Autodesk Inventor part; units mm, degrees
ref_plane "YZ Plane" through (0, 0, 0) normal (1, 0, 0) x (0, 1, 0)
ref_plane "XZ Plane" through (0, 0, 0) normal (0, 1, 0) x (-1, 0, 0)
ref_plane "XY Plane" through (0, 0, 0) normal (0, 0, 1) x (1, 0, 0)
sketch "草图1" plane through (0, 0, 0) normal (0, 1, 0) x (-1, 0, 0)
  line L0 (0, 0) -> (83, 0)
  line L1 (83, 0) -> (83, -124)
  line L2 (83, -124) -> (0, -124)
  line L3 (0, -124) -> (0, 0)
  line L4 (-2, 2) -> (85, 2)
  line L5 (85, 2) -> (85, -126)
  line L6 (85, -126) -> (-2, -126)
  line L7 (-2, -126) -> (-2, 2)
  dimension "d0" = 83
  dimension "d1" = 124
  dimension "d2" = 2
  dimension "d3" = 2
  dimension "d4" = 2
extrude "拉伸1" add sketch "草图1" along normal blind 5 contours L0 L1 L2 L3 | L4 L5 L6 L7
sketch "草图2" plane through (-85, 0, 2) normal (0, 0, 1) x (1, 0, 0)
  line L0 (0, 0) -> (87, 0)
  line L1 (87, 0) -> (87, 5)
  line L2 (0, 5) -> (87, 5)
  line L3 (0, 0) -> (0, 5)
  line L4 (85, 0) -> (2, 0)
  line L5 (8, 0) -> (79, 0)
  line L6 (79, 0) -> (79, 2.5)
  line L7 (79, 2.5) -> (8, 2.5)
  line L8 (8, 2.5) -> (8, 0)
  point P0 (79, 1.25)
  dimension "d8" = 8
  dimension "d9" = 8
extrude "拉伸2" cut sketch "草图2" against normal through all contours L8 L7 L6 L0
sketch "草图3" plane through (2, 0, 2) normal (1, 0, 0) x (0, 0, -1)
  line L0 (2, 0) -> (126, 0)
  line L1 (8, 0) -> (120, 0)
  line L2 (120, 0) -> (120, 2.5)
  line L3 (120, 2.5) -> (8, 2.5)
  line L4 (8, 2.5) -> (8, 0)
  line L5 (0, 0) -> (0, 5)
  line L6 (128, 0) -> (128, 5)
  line L7 (0, 5) -> (128, 5)
  point P0 (8, 1.25)
  point P1 (120, 1.25)
  dimension "d12" = 8
  dimension "d13" = 8
  dimension "d14" = 2.5
extrude "拉伸3" cut sketch "草图3" against normal through all
sketch "草图4" plane through (0, 0, 0) normal (0, -1, 0) x (1, 0, 0)
  line L0 (-6, -6) -> (2, -6)
  line L1 (2, 2) -> (2, -6)
  line L2 (-6, 2) -> (2, 2)
  line L3 (-6, 2) -> (-6, -6)
  line L4 (-6, -6) -> (2, -6)
  line L5 (-77, -126) -> (-77, -118)
  line L6 (-85, 2) -> (-77, 2)
  line L7 (-85, -6) -> (-85, 2)
  line L8 (2, -118) -> (-6, -118)
  line L9 (-85, -126) -> (-85, -118)
  line L10 (-77, -126) -> (-85, -126)
  line L11 (-77, -126) -> (-77, -118)
  line L12 (2, -118) -> (-6, -118)
  line L13 (-6, 2) -> (-6, -6)
  line L14 (2, -126) -> (-6, -126)
  line L15 (2, -118) -> (2, -126)
  line L16 (-6, -118) -> (-6, -126)
  line L17 (-77, -118) -> (-85, -118)
  line L18 (-85, -126) -> (-85, -118)
  line L19 (-77, -126) -> (-85, -126)
  line L20 (-77, -126) -> (-77, -118)
  line L21 (-6, -6) -> (2, -6)
  line L22 (2, 2) -> (2, -6)
  line L23 (-6, 2) -> (2, 2)
  line L24 (-6, -6) -> (2, -6)
  line L25 (-85, 2) -> (-77, 2)
  line L26 (-85, -6) -> (-85, 2)
  line L27 (-6, 2) -> (-6, -6)
  line L28 (2, -126) -> (-6, -126)
  line L29 (2, -118) -> (2, -126)
  line L30 (-77, -118) -> (-85, -118)
  line L31 (-77, -6) -> (-77, 2)
  line L32 (-85, -6) -> (-77, -6)
  line L33 (2, -118) -> (-6, -118)
  line L34 (-85, -126) -> (-85, -118)
  line L35 (-77, -126) -> (-85, -126)
  line L36 (-77, -6) -> (-77, 2)
  line L37 (2, 2) -> (2, -6)
  line L38 (-6, 2) -> (2, 2)
  line L39 (-6, 2) -> (-6, -6)
  line L40 (-85, -6) -> (-77, -6)
  line L41 (-77, -126) -> (-77, -118)
  line L42 (-85, 2) -> (-77, 2)
  line L43 (-85, -6) -> (-85, 2)
  line L44 (2, -118) -> (-6, -118)
  line L45 (-6, -118) -> (-6, -126)
  line L46 (2, -126) -> (-6, -126)
  line L47 (2, -118) -> (2, -126)
  line L48 (-85, -6) -> (-77, -6)
  line L49 (-77, -6) -> (-77, 2)
  line L50 (-85, 2) -> (-77, 2)
  line L51 (-85, -6) -> (-85, 2)
  line L52 (2, 2) -> (2, -6)
  line L53 (-6, 2) -> (2, 2)
  line L54 (-85, -6) -> (-77, -6)
  line L55 (-6, -118) -> (-6, -126)
  line L56 (-77, -118) -> (-85, -118)
  line L57 (-6, -118) -> (-6, -126)
  line L58 (2, -126) -> (-6, -126)
  line L59 (2, -118) -> (2, -126)
  line L60 (-77, -6) -> (-77, 2)
  line L61 (-77, -118) -> (-85, -118)
  line L62 (-85, -126) -> (-85, -118)
  line L63 (-77, -126) -> (-85, -126)
  point P0 (0, 0)
extrude "拉伸4" add sketch "草图4" along normal blind 10
extrude "拉伸5" cut sketch "草图1" along normal blind 43 contours L0 L1 L2 L3
properties part number "底座"
Can you work these out from the model? Positions are in its coordinate system, mm. A direction names the side the tool comes from. Give positions to 0.01 mm unless a question says otherwise; leave off trailing zeros. Write each loop counter-clockwise with the first axis right and the second up, starting at its lowest first coordinate (ties: lowest second). Pieces come first, ordered by that corner, then holes. Notation, with made-up numbers: M -40,-33.75 L 18,-33.75 A15 cw 18,-15.75 Z; hole C 34,-31 d5. An arc over 180 degrees is marked long. Answer in a Markdown table with one row per item. Add a question column.
Item 1: Please list where these lines run through material, in increasing order: L1, parallel to Z at x = -78, y = -2.5; L2, parallel to X at y = 3.5, z = -96.5; L3, parallel to Z at x = -5.5, y = 2.5.
Item 2: Imagine slicing it at C-C, the plane y = -4.25. Write out the boundary of the cut face in (x, z), plus the area to 3 significant figures.
Item 3: Imagine slicing it at A-A, the plane z = -116.5. Write out the boundary of the cut face in (x, y).
Item 4: We'd pull the mould along X, two halves only. Please class faces 4 (the flat face through (0, 4, -63)), 5 (the flat face through (2, 4, -62)), 6 (the flat face through (-2, -10, -122)): released by +X, released by -X, zero draft, split by the parting line, or undercut.
Item 5: For pin 1 Ø1 at (x, z) = (-58, 1) entering from -Y; pin 2 Ø3 at (x, z) = (-4, -120) entering from +Y, each with a flat end and sliding along its axis, tell me the tip position at first contact or that it passes through.
Item 6: Imagine slicing it at B-B, the plane x = -26. Write out the boundary of the cut face in (y, z).
Item 7: On a 3-axis mill with a long thin cutter (end or side, diameter ignored), from which of +Z, -Z, +X, -X, +Y, -Y can I reach the whole of each face in a straight line? I mean faces 1 (the flat face through (-81, -5, -6)), 2 (the flat face through (-6, -5, -122)), 3 (the flat face through (-42, 4, -124)). Say none if no direction works.
Evaluation:
| question | item | result |
|---|---|---|
| 1 | L1 | z = -126 to -118, -6 to 2 |
| 1 | L2 | x = -85 to -83, 0 to 2 |
| 1 | L3 | z = -126 to -124, 0 to 2 |
| 2 | outline | M -85,-126 L -77,-126 L -77,-118 L -85,-118 Z; M -85,-6 L -77,-6 L -77,2 L -85,2 Z; M -6,-126 L 2,-126 L 2,-118 L -6,-118 Z; M -6,-6 L 2,-6 L 2,2 L -6,2 Z |
| 2 | area | 256 mm² |
| 3 | outline | M -85,2.5 L -83,2.5 L -83,5 L -85,5 Z; M 0,2.5 L 2,2.5 L 2,5 L 0,5 Z |
| 4 | face 4 | undercut |
| 4 | face 5 | released by +X |
| 4 | face 6 | zero draft |
| 5 | pin 1 | stops at y = 2.5 |
| 5 | pin 2 | stops at y = 0 |
| 6 | outline | M 2.5,-126 L 5,-126 L 5,-124 L 2.5,-124 Z; M 2.5,0 L 5,0 L 5,2 L 2.5,2 Z |
| 7 | face 1 | +X, -X, -Y |
| 7 | face 2 | +Z, -Z, -Y |
| 7 | face 3 | +Y |
